```python
from build123d import *

# Parameters (mm, degrees)
SKETCH_1_W      = 533.4
SKETCH_1_H      = 360.68
EXTRUDE_1_DEPTH = 12.7
SKETCH_2_W      = 533.4
SKETCH_2_H      = 55.88
EXTRUDE_2_DEPTH = 12.7
CHAMFER1_SIZE   = 7.62
EXTRUDE1_DEPTH  = 12.7
EXTRUDE3_DEPTH  = 12.7


with BuildPart() as part:
    # 草图1 → 凸台-拉伸1 (new body)
    with BuildSketch(Plane(origin=(0, 0, 0), x_dir=(1, 0, 0), z_dir=(0, 1, 0))):
        with Locations((266.7, 180.34)):
            Rectangle(SKETCH_1_W, SKETCH_1_H)
    extrude(amount=EXTRUDE_1_DEPTH)

    # 草图2 → 凸台-拉伸2 (add)
    with BuildSketch(Plane.XY):
        with Locations((266.7, 27.94)):
            Rectangle(SKETCH_2_W, SKETCH_2_H)
    extrude(amount=EXTRUDE_2_DEPTH)

    # Chamfer1
    chamfer1_edges = [part.edges().sort_by_distance(p)[0] for p in [
        (266.7, 0, 12.7),
        (266.7, 55.88, 12.7),
    ]]
    chamfer(chamfer1_edges, length=CHAMFER1_SIZE)

    # Sketch1 → Extrude1 (add)
    with BuildSketch(Plane(origin=(533.4, 0, 0), x_dir=(0, 0, -1), z_dir=(1, 0, 0))):
        Polygon((0, 55.88), (0, 12.7), (43.18, 12.7), align=None)
    extrude(amount=-EXTRUDE1_DEPTH)

    # Sketch4 → Extrude3 (add)
    with BuildSketch(Plane.ZY):
        Polygon((0, 55.88), (0, 12.7), (-43.18, 12.7), align=None)
    extrude(amount=-EXTRUDE3_DEPTH)


solid = part.part
```
The listing builds one solid part. Answer for the finished solid, in the listing's coordinates (mm). A direction names the side the tool comes from. Give positions to 0.01 mm unless a question says otherwise; leave off trailing zeros. Write each loop counter-clockwise with the first axis right and the second up, starting at its lowest first coordinate (ties: lowest second). Pieces come first, ordered by that corner, then holes. Notation, with made-up numbers: (37, 47) -> (74, 47) arc R22 ccw to (74, 82) -> close; hole circle Ø7 at (17, 71). An arc over 180 degrees is marked (long way). Write item = value, one per line. Start each with the question number.
1) Determine the mould class of faces 3 (the face through (533.4, 12, -132)), 4 (the face through (263, 35, 0)), 5 (the face through (263, 28, 12.7)) for opening direction X: +X half, -X half, draft (parallel to the pull), parting line (faces both ways), or undercut.
2) The part is cut by section C-C, the plane z = -256.5. Determine the outline of the cut face in (x, y), and give its area (3 significant figures).
3) Straight lines are drawn through the part: line 1 along X through (y, z) = (17.5, -31); line 2 along Y through (x, z) = (58, -24.5). For each, find the intervals that lie inside material, in ascending order.
4) Which of the six approach directions +Z, -Z, +X, -X, +Y, -Y give full straight-line access (tool end or side, diameter ignored) to faces 1 (the face through (520.7, 25, -12)), 2 (the face through (263, 6, -360.68))?
5) The part is cut by section A-A, the plane y = 18. Determine the outline of the cut face in (x, z), and give its area (3 significant figures).
6) Each of these flat-tipped pins is pushed along its axis until it touches: pin 1 (5 mm diameter, centred on x = 316, z = -221, fed in from +Y); pin 2 (3 mm diameter, centred on x = 324.5, y = 41, fed in from -Z). Where does it stop, or does it pass through?
7) The part is cut by section B-B, the plane x = 113. Determine the outline of the cut face in (y, z), and give its area (3 significant figures).
Solutions:
q1.face_3 = +X half
q1.face_4 = undercut
q1.face_5 = draft
q2.outline = (0, 0) -> (533.4, 0) -> (533.4, 12.7) -> (0, 12.7) -> close
q2.area = 6,770 mm²
q3.line_1 = 0 to 12.7, 520.7 to 533.4
q3.line_2 = 0 to 12.7
q4.face_1 = -Z, +Y
q4.face_2 = -Z, +X, -X, +Y, -Y
q5.outline = (0, -37.88) -> (12.7, -37.88) -> (12.7, 0) -> (520.7, 0) -> (520.7, -37.88) -> (533.4, -37.88) -> (533.4, 12.7) -> (0, 12.7) -> close
q5.area = 7,740 mm²
q6.pin_1 = 12.7
q6.pin_2 = 0
q7.outline = (0, -360.68) -> (12.7, -360.68) -> (12.7, 0) -> (55.88, 0) -> (55.88, 5.08) -> (48.26, 12.7) -> (7.62, 12.7) -> (0, 5.08) -> close
q7.area = 5,230 mm²
